Verification items for the finished model (mm, model axes). A direction names the side the tool comes from. Give positions to 0.01 mm unless a question says otherwise; leave off trailing zeros. Loops run counter-clockwise (first coordinate to the right, second up) from the corner with the lowest first, then second, coordinate; pieces in that order, holes last. Notation, with made-up numbers: M 44,63.25 L 66,63.25 A21 ccw 66,74.25 Z; hole C 40.25,-11.75 d2. An arc over 180 degrees is marked long. Use a Markdown table: item, result.
from build123d import *

# Parameters (mm, degrees)
F0_R     = 1.3
F1_DEPTH = 3.5
F2_T     = -3
F3_SIZE  = 2


with BuildPart() as f1:
    # F0 (on Top) → F1 (new body)
    with BuildSketch(Plane.XY):
        Polygon((-39.15, 34.5), (-43.964466, 34.5), (-47.5, 30.964466), (-47.5, 26.15), (-39.15, 26.15), align=None)
        with Locations((-43.325, 30.325)):
            Circle(F0_R, mode=Mode.SUBTRACT)
        Polygon((-27.15, 34.5), (-39.15, 34.5), (-39.15, 26.15), (-47.5, 26.15), (-47.5, 0), (-47.5, -26.15), (-39.15, -26.15), (-39.15, -32.7), (-39.15, -34.5), (-27.15, -34.5), (27.15, -34.5), (39.15, -34.5), (39.15, -32.7), (39.15, -26.15), (47.5, -26.15), (47.5, 0), (47.5, 26.15), (39.15, 26.15), (39.15, 34.5), (27.15, 34.5), align=None)
        Polygon((43.964466, 34.5), (39.15, 34.5), (39.15, 26.15), (47.5, 26.15), (47.5, 30.964466), align=None)
        with Locations((43.325, 30.325)):
            Circle(F0_R, mode=Mode.SUBTRACT)
        Polygon((-39.15, -26.15), (-47.5, -26.15), (-47.5, -30.964466), (-43.964466, -34.5), (-39.15, -34.5), (-39.15, -32.7), align=None)
        with Locations((-43.325, -30.325)):
            Circle(F0_R, mode=Mode.SUBTRACT)
        Polygon((47.5, -30.964466), (47.5, -26.15), (39.15, -26.15), (39.15, -32.7), (39.15, -34.5), (43.964466, -34.5), align=None)
        with Locations((43.325, -30.325)):
            Circle(F0_R, mode=Mode.SUBTRACT)
    extrude(amount=F1_DEPTH)

    # F2
    f2_openings = [f1.faces().sort_by_distance(p)[0] for p in [
        (0, 0, 3.5),
    ]]
    offset(amount=F2_T, openings=f2_openings)

    # F3
    f3_edges = [f1.edges().sort_by_distance(p)[0] for p in [
        (42.025, 30.325, 0),
        (42.025, -30.325, 0),
        (-44.625, -30.325, 0),
        (-44.625, 30.325, 0),
    ]]
    chamfer(f3_edges, length=F3_SIZE)


solid = f1.part
(1) Cross-section at C-C on x = 34. Record the cut outline in (y, z), then the cut area to 3 significant figures.
Results below:
| item | result |
|---|---|
| outline | M -34.5,0 L 34.5,0 L 34.5,3.5 L 31.5,3.5 L 31.5,3 L -31.5,3 L -31.5,3.5 L -34.5,3.5 Z |
| area | 210 mm^2 |
(2) Gauge pin test, flat ends, axial feed: P1, Ø4, axis at x = 43.325, y = -30.325, coming from the -Z side; P2, Ø10, axis at x = -23, y = 19, coming from the +Z side. Record the tip position at first contact, or that the pin passes through.
Results below:
| item | result |
|---|---|
| P1 | z = 1.3 |
| P2 | z = 3 |
(3) Cross-section at B-B on z = 0.7. Record the cut outline in (x, y) (3 decimals), then the cut area to 3 significant figures.
Results below:
| item | result |
|---|---|
| outline | M -47.5,-30.964 L -43.964,-34.5 L 43.964,-34.5 L 47.5,-30.964 L 47.5,30.964 L 43.964,34.5 L -43.964,34.5 L -47.5,30.964 Z; hole C -43.325,-30.325 d5.2; hole C -43.325,30.325 d5.2; hole C 43.325,-30.325 d5.2; hole C 43.325,30.325 d5.2 |
| area | 6,450 mm^2 |
(4) Cross-section at A-A on y = 4.5. Record the cut outline in (x, z).
Results below:
| item | result |
|---|---|
| outline | M -47.5,0 L 47.5,0 L 47.5,3.5 L 44.5,3.5 L 44.5,3 L -44.5,3 L -44.5,3.5 L -47.5,3.5 Z |
(5) Set-up check for faces 1 (the flat face through (-1, 0, 0)), 2 (the flat face through (-1, 0, 3)): record each of +Z, -Z, +X, -X, +Y, -Y from which the full face is reachable in a straight line by a thin tool's end or side.
Results below:
| item | result |
|---|---|
| face 1 | -Z, +X, -X, +Y, -Y |
| face 2 | +Z |
(6) Material ranges on line 1 (Y direction, x = -42, z = 0.75); line 2 (X direction, y = -30.5, z = 0.5); line 3 (Y direction, x = -10, z = 3.2), recorded low to high.
Results below:
| item | result |
|---|---|
| line 1 | -34.5 to -32.5, -28.15 to 28.15, 32.5 to 34.5 |
| line 2 | -47.5 to -46.12, -40.53 to 40.53, 46.12 to 47.5 |
| line 3 | -34.5 to -31.5, 31.5 to 34.5 |
